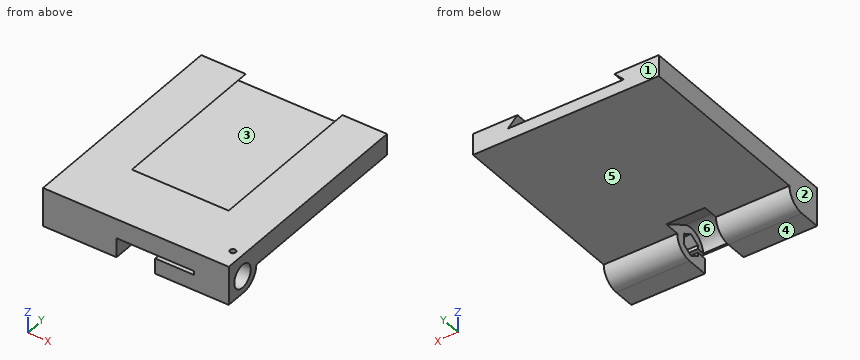
from build123d import *

# Parameters (mm, degrees)
BOSS_EXTRUDE1_DEPTH = 10
BOSS_EXTRUDE3_DEPTH = 10
CUT_EXTRUDE1_DEPTH  = 20
CUT_EXTRUDE2_DEPTH  = 20
SKETCH5_R           = 6
CUT_EXTRUDE3_DEPTH  = 18
SKETCH11_W          = 96
SKETCH11_H          = 11
BOSS_EXTRUDE2_DEPTH = 95
CUT_EXTRUDE10_DEPTH = 20
CUT_EXTRUDE11_DEPTH = 82.75
FILLET3_R           = 9
SKETCH18_R          = 1.5
CUT_EXTRUDE12_DEPTH = 10


with BuildPart() as part:
    # Sketch2 → Boss-Extrude1 (new body)
    with BuildSketch(Plane(origin=(0, 0, 0), x_dir=(1, 0, 0), z_dir=(0, 1, 0))):
        Polygon((-48, 0), (48, 0), (48, 20), (10, 20), (10, 11), (-10, 11), (-10, 20), (-48, 20), align=None)
    extrude(amount=BOSS_EXTRUDE1_DEPTH)

    # Sketch16 → Boss-Extrude3 (add)
    with BuildSketch(Plane.XZ):
        Polygon((-48, 0), (48, 0), (48, -20), (10, -20), (10, -10), (-10, -10), (-10, -20), (-48, -20), align=None)
    extrude(amount=BOSS_EXTRUDE3_DEPTH)

    # Sketch3 → Cut-Extrude1 (cut)
    with BuildSketch(Plane(origin=(-10, 0, 0), x_dir=(0, 0, -1), z_dir=(1, 0, 0))):
        Polygon((16.773502692, 0), (13.886751346, 5), (8.113248654, 5), (5.226497308, 0), (8.113248654, -5), (13.886751346, -5), align=None)
    extrude(amount=-CUT_EXTRUDE1_DEPTH, mode=Mode.SUBTRACT)

    # Sketch4 → Cut-Extrude2 (cut)
    with BuildSketch(Plane.ZY.offset(-10)):
        Polygon((-16.773502692, 0), (-13.886751346, -5), (-12, -5), (-12, -10), (-10, -10), (-10, -5), (-8.113248654, -5), (-5.226497308, 0), (-8.113248654, 5), (-13.886751346, 5), align=None)
    extrude(amount=-CUT_EXTRUDE2_DEPTH, mode=Mode.SUBTRACT)

    # Sketch5 → Cut-Extrude3 (cut)
    with BuildSketch(Plane.ZY.offset(-30)):
        with Locations((-11, 0)):
            Circle(SKETCH5_R)
    extrude(amount=-CUT_EXTRUDE3_DEPTH, mode=Mode.SUBTRACT)

    # Sketch11 → Boss-Extrude2 (add)
    with BuildSketch(Plane(origin=(0, 10, 0), x_dir=(1, 0, 0), z_dir=(0, 1, 0))):
        with Locations((0, 5.5)):
            Rectangle(SKETCH11_W, SKETCH11_H)
    extrude(amount=BOSS_EXTRUDE2_DEPTH)

    # Sketch14 → Cut-Extrude10 (cut)
    with BuildSketch(Plane(origin=(-10, 0, 0), x_dir=(0, 0, -1), z_dir=(1, 0, 0))):
        with BuildLine():
            Line((11, -9), (11, 18))
            Line((11, 18), (3.205771366, 4.5))
            ThreePointArc((3.205771366, 4.5), (3.205771366, -4.5), (11, -9))
        make_face()
    extrude(amount=CUT_EXTRUDE10_DEPTH, mode=Mode.SUBTRACT)

    # Sketch17 → Cut-Extrude11 (cut)
    with BuildSketch(Plane(origin=(0, 105, 0), x_dir=(1, 0, 0), z_dir=(0, 1, 0))):
        Polygon((25, 0), (-25, 0), (-30, 5), (30, 5), align=None)
    extrude(amount=-CUT_EXTRUDE11_DEPTH, mode=Mode.SUBTRACT)

    # Fillet3
    fillet3_edges = [part.edges().sort_by_distance(p)[0] for p in [
        (29, 10, -20),
        (-29, 10, -20),
    ]]
    fillet(fillet3_edges, radius=FILLET3_R - 0.0001)  # a hair under: the kernel refuses the full size

    # Sketch18 → Cut-Extrude12 (cut)
    with BuildSketch(Plane.XY):
        with Locations((43, 0)):
            Circle(SKETCH18_R)
    extrude(amount=-CUT_EXTRUDE12_DEPTH, mode=Mode.SUBTRACT)


solid = part.part
Could you check a few things on this model? Use its own coordinates, in mm. Face numbers are marked on the shaded views. A direction names the side the tool comes from. Coordinates: 2 decimals unless noted, no trailing zeros. Write each loop counter-clockwise with the first axis right and the second up, starting at its lowest first coordinate (ties: lowest second). Pieces come first, ordered by that corner, then holes. Notation, with made-up numbers: (14.5, -29) - (39.5, -29) arc R29 ccw to (39.5, -1) - close; hole circle Ø6 at (74.5, -5.5). An arc over 180 degrees is marked (long way). Write item = value, one per line.
1) We'd pull the mould along X, two halves only. Please class the marked faces 1, 2 and 3: +X half, -X half, draft (parallel to the pull), parting line (faces both ways), or undercut.
Result set:
face_1 = draft
face_2 = -X half
face_3 = undercut
2) Will these pins go through, and if not, where does the flat tip stop? pin 1 Ø6.5 at (x, z) = (20.5, -11) entering from -Y; pin 2 Ø6 at (x, y) = (18.5, 45.5) entering from +Z; pin 3 Ø12 at (x, y) = (-8, 9) entering from -Z; pin 4 Ø0.9 at (x, z) = (23.5, -13) entering from +Y.
Result set:
pin_1 = -10
pin_2 = -5
pin_3 = -19.69
pin_4 = 9.87
3) For the marked faces 4, 5 and 6, which set-ups out of +Z, -Z, +X, -X, +Y, -Y let a thin tool reach every point of the face, with its end or its side?
Result set:
face_4 = -Z, +X, -X, +Y, -Y
face_5 = -Z, +X, -X, +Y
face_6 = -Z
4) Suppose I cut it at B-B on y = 97. Please give me the cut outline in (x, z), plus the area to 3 significant figures.
Result set:
outline = (-48, -11) - (48, -11) - (48, 0) - (25, 0) - (30, -5) - (-30, -5) - (-25, 0) - (-48, 0) - close
area = 781 mm2
5) Please list where these lines run through material, in increasing order: line 1 (X direction, y = 0, z = -3.8); line 2 (X direction, y = 0, z = -1.3); line 3 (X direction, y = 2, z = -4). Write a range as [from, to].
Result set:
line_1 = [-48, -10], [10, 41.5], [44.5, 48]
line_2 = [-48, 41.5], [44.5, 48]
line_3 = [-48, -10], [10, 48]
